Autodesk Inventor part; units mm, degrees
ref_plane "Arbeitsebene1" through (0, 0, -7.5) normal (0, 0, 1) x (1, 0, 0)
ref_plane "YZ Plane" through (0, 0, 0) normal (1, 0, 0) x (0, 1, 0)
ref_plane "XZ Plane" through (0, 0, 0) normal (0, 1, 0) x (-1, 0, 0)
sketch "Skizze1" plane through (0, 0, 0) normal (0, 0, 1) x (1, 0, 0)
  line L0 (6.45, 0) -> (15, 0)
  line L1 (15, 0) -> (15, 30)
  line L2 (15, 30) -> (0, 30)
  line L3 (0, 30) -> (0, 3.0582)
  arc A0 (6.45, 0) -> (0, 3.0582) centre (2.5, 0) ccw
  line L4 (-3, 0) -> (18, 0)
  line L5 (0, -6) -> (0, 36)
  point P0 (0, 0)
  dimension "d0" = 30
  dimension "d1" = 15
  dimension "d2" = 7.9
  dimension "d3" = 2.5
extrude "Extrusion1" add sketch "Skizze1" along normal mid plane 17.5 contours A0 L3 L2 L1 L0
ref_plane "Arbeitsebene1" through (0, 0, -7.5) normal (0, 0, 1) x (1, 0, 0)
sketch "Skizze2" plane through (0, 0, -7.5) normal (0, 0, 1) x (1, 0, 0)
  circle A0 centre (2.5, 0) radius 3.95
  arc A1 (6.45, 0) -> (0, 3.0582) centre (2.5, 0) ccw
  circle A2 centre (2.5, 0) radius 3.45
  line L0 (0, 3.0582) -> (0, 2.3775)
  line L1 (15, 0) -> (6.45, 0)
  line L2 (6.45, 0) -> (5.95, 0)
  point P0 (0, 0)
  point P1 (0, 3.0582)
  dimension "d7" = 7.9
  dimension "d8" = 6.9
extrude "Extrusion2" add sketch "Skizze2" along normal up to surface (16.25 mm away) contours L2 A2 L0 A0 picked at (6.25, 0.2945)
sketch "Skizze3" plane through (15, 0, 8.75) normal (1, 0, 0) x (0, 0, -1)
  line L0 (17.5, 30) -> (17.5, 0)
  line L1 (-3.5, 0) -> (21, 0)
  point P0 (8.75, 0)
  point P1 (14.5, 20.5)
  point P2 (14.5, 6)
  dimension "d11" = 3
  dimension "d12" = 3
  dimension "d13" = 6
  dimension "d14" = 14.5
hole "Bohrung1" at (15, 20.5, -5.75) at (15, 6, -5.75) direction (-1, 0, 0) diameter 3.242 depth 8 tip angle 118
sketch "Skizze4" plane through (6.45, 0, -8.75) normal (0, -1, 0) x (1, 0, 0)
  line L0 (-9.45, 8.75) -> (11.55, 8.75)
  line L1 (8.55, 0) -> (8.55, 17.5)
  line L2 (8.55, 17.5) -> (-0.5, 17.5)
  line L3 (-6.45, 21) -> (-6.45, -3.5)
  point P0 (-6.45, 8.75)
  point P1 (5.5, 14.5)
  point P2 (5.5, 8.75)
  dimension "d24" = 3
  dimension "d35" = 11.95
hole "Bohrung2" at (11.95, 0, 5.75) at (11.95, 0, 0) direction (0, 1, 0) diameter 4 depth 6 tip angle 118
sketch "Skizze5" plane through (0, 0, 8.75) normal (0, 0, 1) x (1, 0, 0)
  circle A0 centre (2.5, 0) radius 6
  arc A1 (5.95, 0) -> (0, 2.3775) centre (2.5, 0) ccw
  line L0 (0, 2.3775) -> (0, 5.4544)
  line L1 (5.95, 0) -> (8.5, 0)
  line L2 (15, 0) -> (5.95, 0)
  point P0 (0, 0)
  dimension "d32" = 12
extrude "Extrusion3" cut sketch "Skizze5" against normal blind 14 contours L1 A1 L0 A0 picked at (7.6008, 0.4409)
chamfer "Fasen1" distance 2 angle 45 1 edges at (3.7801, 3.2037, -5.25)
sketch "Skizze6" plane through (0, 30, 8.75) normal (0, 1, 0) x (1, 0, 0)
  line L0 (0, 17.5) -> (15, 17.5)
  line L1 (0, 17.5) -> (0, 0)
  point P0 (0, 8.75)
  point P1 (10, 5)
  point P2 (10, 13)
  point P3 (3, 9)
  dimension "d39" = 4.5
  dimension "d40" = 12.5
  dimension "d41" = 8.5
  dimension "d42" = 10
  dimension "d43" = 3
hole "Bohrung3" [suppressed]
hole "Bohrung4" [suppressed]
equation "\"d0\" = Laenge_Grundkoerper"
equation "\"d1\" = Breite_Grundkoerper"
equation "\"d2\" = D_Scheibe"
equation "\"d3\" = Abstand_D_Scheibe"
equation "\"d4\" = Tiefe_Grundkoerper"
equation "\"d7\" = D_Scheibe"
equation "\"d9\" = Tiefe_Grundkoerper"
equation "\"d25\" = D_Zentrierbohrung"
equation "\"d30\" = T_Zentrierbohrung"
equation "\"Laenge_Grundkoerper\" = 30"
equation "\"Breite_Grundkoerper\" = 15"
equation "\"D_Scheibe\" = 7.9"
equation "\"Abstand_D_Scheibe\" = 2.5"
equation "\"Abstand_Arbeitsebene\" = 2"
equation "\"Tiefe_Grundkoerper\" = 17.5"
equation "\"Abstand_Bohrungen_y\" = 3"
equation "\"Abstand_Bohrungen_x\" = 6"
equation "\"Abstand_Bohrungen\" = 14.5"
equation "\"Zentrierbohrung_x\" = 6"
equation "\"D_Zentrierbohrung\" = 4"
equation "\"T_Zentrierbohrung\" = 6"
equation "\"Zentrierbohrung_y\" = 3"
properties part number "JH_int_Greiferkoerper"
Build history of the part. All positions in model axes, mm. A direction names the side the tool comes from. Coordinates: 2 decimals unless noted, no trailing zeros. One line per item, written item: value.
(1) Drop flat-ended pins along their axis: pin 1 Ø3 at (x, z) = (11.95, 0) entering from -Y; pin 2 Ø1.8 at (x, y) = (3, 4) entering from +Z. Give the stop position or say it passes through.
Checked values:
pin 1: y = 6.3
pin 2: z = -5.77
(2) Slice it at A-A, the plane x = 7.5. Count the separate pieces of the cut face and the enclosed holes in it, plus the area to 3 significant figures.
Checked values:
separate pieces: 1
enclosed holes: 2
area: 461 mm2
(3) Tool access for faces 5 (the cylindrical face through (10.944, 7.582, -5.399)), 6 (the cylindrical face through (4.136, 3.595, -8.134)), 7 (the flat face through (7, 15, 8.75)), 8 (the flat face through (5.5, 4.8, -5.25)), 9 (the cylindrical face through (13.902, 3.042, 0.434)): list every direction of +Z, -Z, +X, -X, +Y, -Y with a clear straight run to the whole face (end or side of a thin tool).
Checked values:
face 5: +X
face 6: -Z, -Y
face 7: +Z, +X, -X, +Y, -Y
face 8: +Z, -Y
face 9: -Y
(4) Mould opens along Y. For faces 1 (the flat face through (15, 15, 0)), 2 (the flat face through (11, 0, -2)), 3 (the conical face through (6.195, 20.69, -5.543)), 4 (the conical face through (6.195, 6.012, -5.469)) say: pulls with the +Y half, pulls with the -Y half, needs draft (parallel to the pull), parting line crosses it, or undercut.
Checked values:
face 1: needs draft
face 2: pulls with the -Y half
face 3: undercut
face 4: undercut
(5) Probe line 1 (Z direction, x = 11.95, y = 1.7); line 2 (Y direction, x = 12, z = -5.75); line 3 (Y direction, x = 7.5, z = -6.5). List the from-to ranges inside material, lowest first. Write a range as [from, to].
Checked values:
line 1: [-8.75, -2], [2, 3.75], [7.75, 8.75]
line 2: [0, 4.38], [7.62, 18.88], [22.12, 30]
line 3: [0, 4.56], [7.44, 19.06], [21.94, 30]
